Check sheet for the modelled part. Datum: model origin and axes. Units: mm. A direction names the side the tool comes from. Give positions to 0.01 mm unless a question says otherwise; leave off trailing zeros. Loops run counter-clockwise (first coordinate to the right, second up) from the corner with the lowest first, then second, coordinate; pieces in that order, holes last. Notation, with made-up numbers: M -29,18 L 17,18 A26 ccw 17,46 Z; hole C -26,56 d10. An arc over 180 degrees is marked long. Use one line per item in the form item = value.
Autodesk Inventor part; units mm, degrees
ref_plane "YZ Plane" through (0, 0, 0) normal (1, 0, 0) x (0, 1, 0)
ref_plane "XZ Plane" through (0, 0, 0) normal (0, 1, 0) x (-1, 0, 0)
ref_plane "XY Plane" through (0, 0, 0) normal (0, 0, 1) x (1, 0, 0)
sketch "Эскиз1" plane through (0, 0, 0) normal (0, 0, 1) x (1, 0, 0)
  line L0 (-7, -3.5) -> (7, -3.5) construction
  line L1 (7, -3.5) -> (7, 3.5)
  line L2 (7, 3.5) -> (-7, 3.5)
  line L3 (-7, 3.5) -> (-7, -3.5)
  line L4 (-7, -3.5) -> (7, 3.5) construction
  line L5 (7, -3.5) -> (-7, 3.5) construction
  line L6 (0, -3.5) -> (0, -12.5) construction
  line L7 (-7, -3.5) -> (-3.289, -13.697)
  line L8 (7, -3.5) -> (3.289, -13.697)
  arc A0 (-3.289, -13.697) -> (3.289, -13.697) centre (0, -12.5) ccw
  point P0 (0, 0)
  point P1 (0, 0)
  point P2 (0, 0)
  point P3 (0, 0)
  dimension "d0" = 14
  dimension "d1" = 7
  dimension "d4" = 9
  dimension "d5" = 3.5
extrude "Выдавливание1" add sketch "Эскиз1" along normal blind 1.5
sketch "Эскиз4" plane through (0, 0, 1.5) normal (0, 0, 1) x (1, 0, 0)
  line L0 (7, 3.5) -> (-7, 3.5)
  line L1 (7, -3.5) -> (7, 3.5)
  line L2 (-7, 3.5) -> (-7, -3.5)
  line L3 (-7, -3.5) -> (7, -3.5)
  point P0 (0, 0)
extrude "Выдавливание6" add sketch "Эскиз4" along normal blind 2.9
sketch "Эскиз2" plane through (0, 0, 1.5) normal (0, 0, 1) x (1, 0, 0)
  arc A0 (-3.289, -13.697) -> (3.289, -13.697) centre (0, -12.5) ccw construction
  circle A1 centre (0, -12.5) radius 1.25
  point P0 (0, 0)
  dimension "d8" = 2.5
extrude "Выдавливание9" add sketch "Эскиз2" along normal blind 5
fillet "Сопряжение1" radius 3.5 2 edges at (7, 3.5, 2.2) (-7, 3.5, 2.2)
sketch "Эскиз5" plane through (0, 0, 4.4) normal (0, 0, 1) x (1, 0, 0)
  circle A0 centre (0, -9.5) radius 1.5 construction
  line L0 (7, -3.5) -> (-7, -3.5) construction
  line L1 (0, -3.5) -> (0, 3.5) construction
  line L2 (-7, 3.5) -> (7, 3.5) construction
  circle A1 centre (3.5, 0) radius 0.5
  line L3 (3.5, 3.5) -> (3.5, 0) construction
  line L4 (3.5, 0) -> (0, 0) construction
  circle A2 centre (-3.5, 0) radius 0.5
  dimension "d34" = 1
hole "Отверстие1" at (-3.5, 0, 4.4) at (3.5, 0, 4.4) direction (0, 0, -1) diameter 1 end through all countersink diameter 1.5 countersink angle 90
properties part number "переходник"
1) Section check D-D (y = -2). Record the cut outline in (x, z).
Evaluation:
outline = M -7,0 L 7,0 L 7,4.4 L -7,4.4 Z
2) Set-up check for faces 1 (the face through (-0.16, -13.74, 3.96)), 2 (the face through (0, 0, 4.4)), 3 (the face through (5, -9, 1)): record each of +Z, -Z, +X, -X, +Y, -Y from which the full face is reachable in a straight line by a thin tool's end or side.
Evaluation:
face_1 = +Z
face_2 = +Z, +X, -X, +Y
face_3 = +Z, -Z, +X, -Y
3) Scan lines: line 1 (X direction, y = 0, z = 1.15); line 2 (Y direction, x = 3.5, z = 2); line 3 (Z direction, x = -0.75, y = -4). Record each from-to range of solid material in increasing order.
Evaluation:
line_1 = -7 to -4, -3 to 3, 4 to 7
line_2 = -3.5 to -0.5, 0.5 to 3.5
line_3 = 0 to 1.5
4) Section check B-B (x = 0). Record the cut outline in (y, z), then the cut area to 4 significant figures.
Evaluation:
outline = M -16,0 L 3.5,0 L 3.5,4.4 L -3.5,4.4 L -3.5,1.5 L -11.25,1.5 L -11.25,6.5 L -13.75,6.5 L -13.75,1.5 L -16,1.5 Z
area = 62.05 mm^2
5) Section check C-C (z = 1). Record the cut outline in (x, y).
Evaluation:
outline = M -7,-3.5 L -3.29,-13.7 A3.5 ccw 3.29,-13.7 L 7,-3.5 L 7,0 A3.5 ccw 3.5,3.5 L -3.5,3.5 A3.5 ccw -7,0 Z; hole C -3.5,0 d1; hole C 3.5,0 d1
6) Depth check by flat-ended pin: pin 1 Ø7.5 at (x, y) = (-2.5, 0.5) entering from +Z; pin 2 Ø2 at (y, z) = (-12.5, 2) entering from -X; pin 3 Ø1.5 at (x, z) = (3.5, 2.5) entering from -Y; pin 4 Ø2 at (y, z) = (-2, 5.5) entering from +X. Enter the tip coordinate at first touch or a pass-through.
Evaluation:
pin_1 = 4.4
pin_2 = -4.04
pin_3 = -3.5
pin_4 = through
7) Section check A-A (z = 2.5). Record the cut outline in (x, y), then the cut area to 3 significant figures.
Evaluation:
outline = M -7,-3.5 L 7,-3.5 L 7,0 A3.5 ccw 3.5,3.5 L -3.5,3.5 A3.5 ccw -7,0 Z; C 0,-12.5 d2.5; hole C -3.5,0 d1; hole C 3.5,0 d1
area = 96.1 mm^2
8) Release check for a two-part mould opening along X. For faces 4 (the face through (-4, 0, 2)), 5 (the face through (0, -16, 1)), 6 (the face through (0, -12, 6.5)) record: pulls with the +X half, pulls with the -X half, needs draft (parallel to the pull), parting line crosses it, or undercut.
Evaluation:
face_4 = undercut
face_5 = parting line crosses it
face_6 = needs draft
